from build123d import *

# Parameters (mm, degrees)
SKETCH4_W                  = 106
SKETCH4_H                  = 30
BOSS_EXTRUDE2_DEPTH        = 13
M4X0_7_TAPPED_HOLE1_D      = 3.3
SKETCH28_W                 = 106
SKETCH28_H                 = 4.5
BOSS_EXTRUDE3_DEPTH        = 43.5
SKETCH32_W                 = 43.5
SKETCH32_H                 = 4.5
BOSS_EXTRUDE10_DEPTH       = 5
F_8_0_199_DIAMETER_HOLE1_D = 5.0546
SKETCH44_W                 = 107.027081708
SKETCH44_H                 = 13.5
BOSS_EXTRUDE17_DEPTH       = 13
M4X0_7_TAPPED_HOLE2_D      = 3.3


with BuildPart() as part:
    # Sketch4 → Boss-Extrude2 (new body)
    with BuildSketch(Plane.XY):
        with Locations((-36.891047602, -35.322762913)):
            Rectangle(SKETCH4_W, SKETCH4_H)
    extrude(amount=-BOSS_EXTRUDE2_DEPTH)

    # M4x0.7 Tapped Hole1 (through all)
    with Locations(Plane(origin=(-74.390985602, -20.322762913, -4.15), x_dir=(0, 0, 1), z_dir=(0, 1, 0))):
        with Locations((0, 0), (0, 25), (-0.055677319, 74.999938), (0, 50)):
            Hole(M4X0_7_TAPPED_HOLE1_D / 2)

    # Sketch28 → Boss-Extrude3 (add)
    with BuildSketch(Plane.XY):
        with Locations((-36.891047602, -48.072762913)):
            Rectangle(SKETCH28_W, SKETCH28_H)
    extrude(amount=BOSS_EXTRUDE3_DEPTH)

    # Sketch32 → Boss-Extrude10 (add)
    with BuildSketch(Plane.ZY.offset(89.891047602)):
        with Locations((21.75, -48.072762913)):
            Rectangle(SKETCH32_W, SKETCH32_H)
    extrude(amount=BOSS_EXTRUDE10_DEPTH)

    # #8 (0.199) Diameter Hole1 (through all)
    with Locations(Plane(origin=(-80.669073904, -45.822762913, 16.25), x_dir=(0, 0, 1), z_dir=(0, 1, 0))):
        with Locations((0, 0), (0, 91.778026302), (0, 81.778026302), (0, 10)):
            Hole(F_8_0_199_DIAMETER_HOLE1_D / 2)

    # Sketch44 → Boss-Extrude17 (add)
    with BuildSketch(Plane(origin=(0, -45.822762913, 0), x_dir=(1, 0, 0), z_dir=(0, 1, 0))):
        with Locations((-37.404588456, -36.75)):
            Rectangle(SKETCH44_W, SKETCH44_H)
    extrude(amount=BOSS_EXTRUDE17_DEPTH)

    # M4x0.7 Tapped Hole2 (through all)
    with Locations(Plane(origin=(-74.391047602, -32.822762913, 34.71), x_dir=(0, 0, 1), z_dir=(0, 1, 0))):
        with Locations((0, 0), (0, 25), (0, 50), (0, 75)):
            Hole(M4X0_7_TAPPED_HOLE2_D / 2)


solid = part.part
Read the model definition and answer for the solid it produces. Units are mm, in the model's axes. A direction names the side the tool comes from. Coordinates: 2 decimals unless noted, no trailing zeros. Loops run counter-clockwise (first coordinate to the right, second up) from the corner with the lowest first, then second, coordinate; pieces in that order, holes last. Notation, with made-up numbers: (70.5, -3.5) -> (79.5, -3.5) arc R17 cw to (79.5, 5.5) -> close; hole circle Ø1 at (-11.75, -9.5). An arc over 180 degrees is marked (long way). Answer in a Markdown table with one row per item.
Item 1: A cutting plane is placed at D-D on z = -4. Determine the outline of the cut face in (x, y).
Returned:
| item | result |
|---|---|
| outline | (-89.89, -50.32) -> (-76.03, -50.32) -> (-76.03, -20.32) -> (-89.89, -20.32) -> close; (-72.75, -50.32) -> (-51.03, -50.32) -> (-51.03, -20.32) -> (-72.75, -20.32) -> close; (-47.75, -50.32) -> (-26.03, -50.32) -> (-26.03, -20.32) -> (-47.75, -20.32) -> close; (-22.75, -50.32) -> (-1.03, -50.32) -> (-1.03, -20.32) -> (-22.75, -20.32) -> close; (2.25, -50.32) -> (16.11, -50.32) -> (16.11, -20.32) -> (2.25, -20.32) -> close |
Item 2: A cutting plane is placed at A-A on z = 16.25. Determine the outline of the cut face in (x, y).
Returned:
| item | result |
|---|---|
| outline | (-94.89, -50.32) -> (-83.2, -50.32) -> (-83.2, -45.82) -> (-94.89, -45.82) -> close; (-78.14, -50.32) -> (-73.2, -50.32) -> (-73.2, -45.82) -> (-78.14, -45.82) -> close; (-68.14, -50.32) -> (-1.42, -50.32) -> (-1.42, -45.82) -> (-68.14, -45.82) -> close; (3.64, -50.32) -> (8.58, -50.32) -> (8.58, -45.82) -> (3.64, -45.82) -> close; (13.64, -50.32) -> (16.11, -50.32) -> (16.11, -45.82) -> (13.64, -45.82) -> close |
Item 3: Each of these flat-tipped pins is pushed along its axis until it touches: P1, Ø5.5, axis at x = -24.39, z = -4.15, coming from the -Y side; P2, Ø7, axis at x = -30.5, z = 36, coming from the +Y side; P3, Ø8, axis at x = -39.5, z = 8, coming from the +Y side; P4, Ø6, axis at x = -73.5, y = -29.5, coming from the +Z side. Where does it stop, or does it pass through?
Returned:
| item | result |
|---|---|
| P1 | stops at y = -50.32 |
| P2 | stops at y = -32.82 |
| P3 | stops at y = -45.82 |
| P4 | stops at z = 0 |
Item 4: A cutting plane is placed at C-C on x = -87. Determine the outline of the cut face in (y, z), plus the area to 3 significant figures.
Returned:
| item | result |
|---|---|
| outline | (-50.32, -13) -> (-20.32, -13) -> (-20.32, 0) -> (-45.82, 0) -> (-45.82, 30) -> (-32.82, 30) -> (-32.82, 43.5) -> (-50.32, 43.5) -> close |
| area | 761 mm^2 |
Item 5: For faces 5 (the flat face through (-38, -35, -13)), 6 (the flat face through (-38, -39, 30)), 7 (the flat face through (-89.891, -36, -7)), 8 (the flat face through (-38, -32.823, 37)), 9 (the flat face through (-94.891, -48, 21)), determine the directions among +Z, -Z, +X, -X, +Y, -Y from which every point of the face is accessible in a straight line to the end or side of a thin tool.
Returned:
| item | result |
|---|---|
| face 5 | -Z, +X, -X, +Y, -Y |
| face 6 | +X, -X, +Y |
| face 7 | -Z, -X, +Y, -Y |
| face 8 | +Z, +X, -X, +Y |
| face 9 | +Z, -Z, -X, +Y, -Y |
Item 6: Straight lines are drawn through the part: line 1 along X through (y, z) = (-46, 34.71); line 2 along X through (y, z) = (-34.5, 35); line 3 along Z through (x, y) = (-74.5, -36). For each, find the intervals that lie inside material, in ascending order. Write a range as [from, to].
Returned:
| item | result |
|---|---|
| line 1 | x = [-94.89, -76.04], [-72.74, -51.04], [-47.74, -26.04], [-22.74, -1.04], [2.26, 16.11] |
| line 2 | x = [-90.92, -76.02], [-72.77, -51.02], [-47.77, -26.02], [-22.77, -1.02], [2.23, 16.11] |
| line 3 | z = [-13, -5.8], [-2.5, 0], [30, 33.06], [36.36, 43.5] |
Item 7: A cutting plane is placed at B-B on y = -40. Give the number of separate pieces and of enclosed holes in the cut face, plus the area to 3 significant figures.
Returned:
| item | result |
|---|---|
| separate pieces | 2 |
| enclosed holes | 8 |
| area | 2,750 mm^2 |
Item 8: For a pull along Z with two mould halves and no side action, classify faces 1 (the flat face through (-90.918, -39, 37)), 2 (the flat face through (-92, -48, 0)), 3 (the cylindrical face through (-0.023, -41.695, 33.186)), 4 (the flat face through (-40, -42, 43.5)) as released by +Z, released by -Z, zero draft, split by the parting line, or undercut.
Returned:
| item | result |
|---|---|
| face 1 | zero draft |
| face 2 | released by -Z |
| face 3 | undercut |
| face 4 | released by +Z |
